Source: three-view drawing plus pictorial views. Frame: mm from the lowest corner of the part. A direction names the side the tool comes from. Round coordinates to 2 decimals unless told otherwise and drop trailing zeros. Loops run counter-clockwise (first coordinate to the right, second up) from the corner with the lowest first, then second, coordinate; pieces in that order, holes last. Notation, with made-up numbers: (69, 6) -> (128, 6) arc R16 cw to (128, 21) -> close; hole circle Ø6 at (16, -22). An arc over 180 degrees is marked (long way). Answer in a Markdown table with one row per item. Add a question column.
Q1. Section A-A, the plane y = 20. Output: boundary loops of the cut face in (x, z).
Q2. Reachability of the marked faces 1 and 2 from +Z, -Z, +X, -X, +Y, -Y: full face, straight path, thin tool, end or side. Return the list, or none.
Q3. Pin query (flat end, axial travel): pin 1 (5 mm diameter, centred on y = 19, z = 7.5, fed in from -X); pin 2 (1.5 mm diameter, centred on x = 25.5, z = 4, fed in from -Y); pin 3 (1 mm diameter, centred on y = 32.5, z = 7.5, fed in from +X). Return the tip coordinate at first contact, or that it passes through.
Q4. Section C-C, the plane z = 0.75. Output: boundary loops of the cut face in (x, y).
Q5. Ray query, L1, parallel to Y at x = 20, z = 3.75; L2, parallel to Y at x = 20, z = 2; L3, parallel to Z at x = 27.5, y = 7. Return the intervals inside material, ascending. Write a range as from..to.
Q6. Section D-D, the plane y = 9.5. Output: boundary loops of the cut face in (x, z), and give its area (3 significant figures).
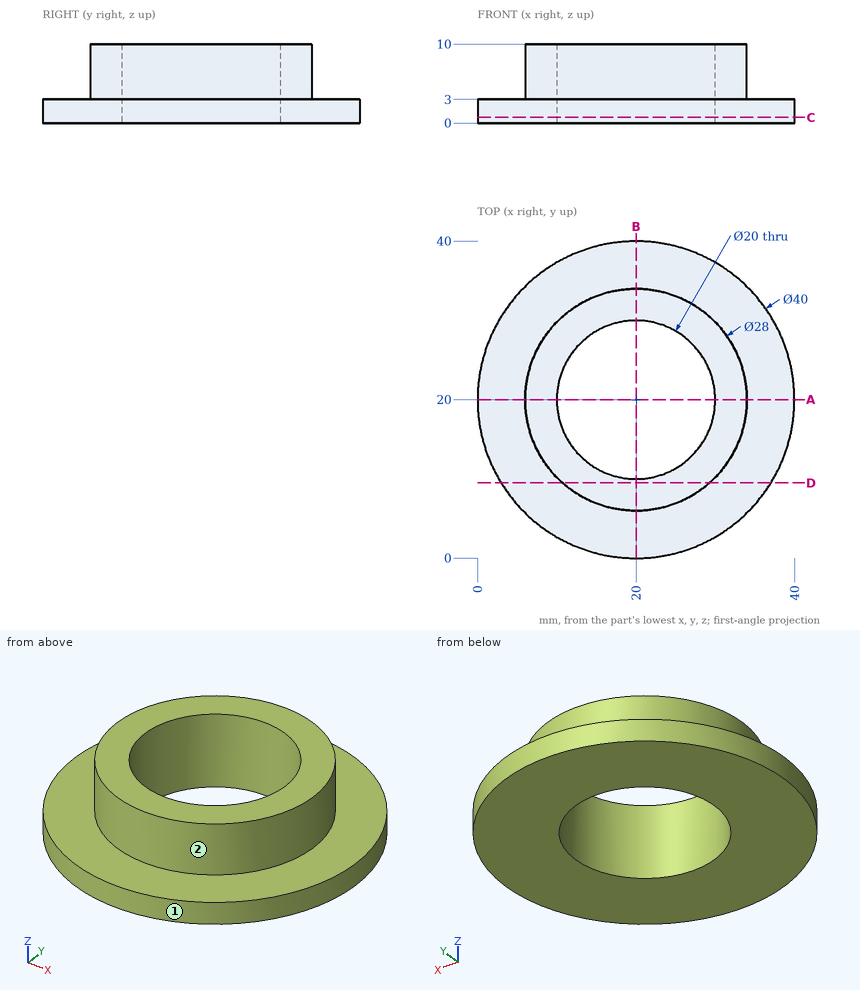
Answer block:
| question | item | result |
|---|---|---|
| 1 | outline | (0, 0) -> (10, 0) -> (10, 10) -> (6, 10) -> (6, 3) -> (0, 3) -> close; (30, 0) -> (40, 0) -> (40, 3) -> (34, 3) -> (34, 10) -> (30, 10) -> close |
| 2 | face 1 | +Z, -Z |
| 2 | face 2 | +Z |
| 3 | pin 1 | x = 6 |
| 3 | pin 2 | y = 6.83 |
| 3 | pin 3 | x = 27.21 |
| 4 | outline | circle Ø40 at (20, 20); hole circle Ø20 at (20, 20) |
| 5 | L1 | 6..10, 30..34 |
| 5 | L2 | 0..10, 30..40 |
| 5 | L3 | 0..3 |
| 6 | outline | (2.98, 0) -> (37.02, 0) -> (37.02, 3) -> (29.26, 3) -> (29.26, 10) -> (10.74, 10) -> (10.74, 3) -> (2.98, 3) -> close |
| 6 | area | 232 mm^2 |
